Check sheet for the modelled part. Datum: model origin and axes. Units: mm. Face numbers are marked on the shaded views. A direction names the side the tool comes from. Coordinates: 2 decimals unless noted, no trailing zeros. Loops run counter-clockwise (first coordinate to the right, second up) from the corner with the lowest first, then second, coordinate; pieces in that order, holes last. Notation, with made-up numbers: (65, 29) - (121, 29) arc R29 ccw to (121, 56) - close; hole circle Ø9 at (75, 89). An arc over 180 degrees is marked (long way). Use a Markdown table: item, result. Add a question column.
1) Sectioned sample at C-C, the plane z = 11. Enter the section's corners in (x, y), then the cut area to 3 significant figures.
2) Tool access check on the marked faces 1, 2 and 3. Record the directions out of +Z, -Z, +X, -X, +Y, -Y that give a thin tool (end or side, any length) a straight path to the whole face; none if there is none.
3) Sectioned sample at A-A, the plane z = 0. Enter the section's corners in (x, y), then the cut area to 3 significant figures.
4) Sectioned sample at D-D, the plane z = -15. Enter the section's corners in (x, y).
5) Thickness scan on line 1 (X direction, y = 17, z = -5); line 2 (Z direction, x = 8.5, y = 17); line 3 (Y direction, x = 13.5, z = 1.5). Record the ranges inside material, lowest first.
6) Sectioned sample at B-B, the plane x = 13.5. Enter the section's corners in (y, z).
7) Go/stop test with flat-tipped pins: P1, Ø10, axis at x = 13, z = 8.5, coming from the +Y side; P2, Ø2, axis at x = 0, z = 10.5, coming from the -Y side; P3, Ø2, axis at x = 9.53, z = -5.5, coming from the -Y side. Record where each tip stops, or that it passes through.
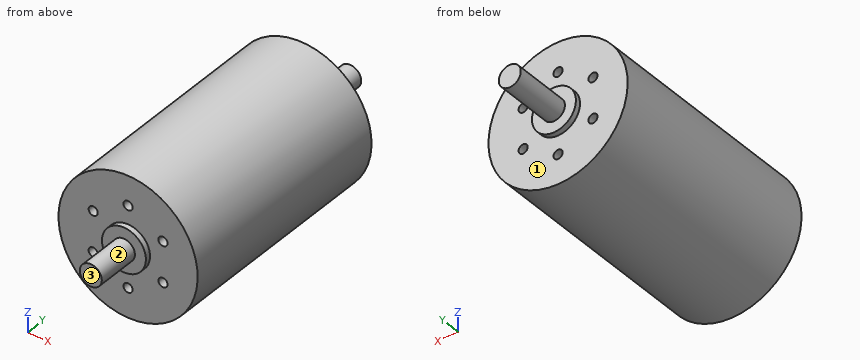
from build123d import *

# Parameters (mm, degrees)
ESQUISSE2_R             = 1.25
ENL_V_MAT_EXTRU_1_DEPTH = 5
ENL_V_START             = -58
ESQUISSE2_2_R           = 1.25
ENL_V_MAT_EXTRU_2_DEPTH = 5


with BuildPart() as part:
    # Esquisse1 → Révolution1 (revolve)
    with BuildSketch(Plane.XY, mode=Mode.PRIVATE) as r_volution1_sk:
        Polygon((0, 0), (0, 94), (3, 94), (3, 78), (6, 78), (6, 76.5), (19, 76.5), (19, 13.5), (6, 13.5), (6, 12), (3, 12), (3, 0), align=None)
    revolve(r_volution1_sk.sketch.rotate(Axis((0, 0, 0), (0, 1, 0)), 90), axis=Axis((0, 0, 0), (0, 1, 0)))

    # Esquisse2 → Enlèv. mat.-Extru.1 (cut)
    with BuildSketch(Plane(origin=(0, 76.5, 0), x_dir=(1, 0, 0), z_dir=(0, 1, 0))):
        with Locations(Location((0, 11, 0), (0, 0, 270))):
            Circle(ESQUISSE2_R)
        with Locations(Location((9.526279442, 5.5, 0), (0, 0, 270))):
            Circle(ESQUISSE2_R)
        with Locations(Location((9.526279442, -5.5, 0), (0, 0, 270))):
            Circle(ESQUISSE2_R)
        with Locations(Location((0, -11, 0), (0, 0, 270))):
            Circle(ESQUISSE2_R)
        with Locations(Location((-9.526279442, -5.5, 0), (0, 0, 270))):
            Circle(ESQUISSE2_R)
        with Locations(Location((-9.526279442, 5.5, 0), (0, 0, 270))):
            Circle(ESQUISSE2_R)
    extrude(amount=-ENL_V_MAT_EXTRU_1_DEPTH, mode=Mode.SUBTRACT)

    # Esquisse2<2> → Enlèv. mat.-Extru.2 (cut)
    with BuildSketch(Plane(origin=(0, 76.5, 0), x_dir=(1, 0, 0), z_dir=(0, 1, 0)).offset(ENL_V_START)):
        with Locations(Location((0, 11, 0), (0, 0, 270))):
            Circle(ESQUISSE2_2_R)
        with Locations(Location((9.526279442, 5.5, 0), (0, 0, 270))):
            Circle(ESQUISSE2_2_R)
        with Locations(Location((9.526279442, -5.5, 0), (0, 0, 270))):
            Circle(ESQUISSE2_2_R)
        with Locations(Location((0, -11, 0), (0, 0, 270))):
            Circle(ESQUISSE2_2_R)
        with Locations(Location((-9.526279442, -5.5, 0), (0, 0, 270))):
            Circle(ESQUISSE2_2_R)
        with Locations(Location((-9.526279442, 5.5, 0), (0, 0, 270))):
            Circle(ESQUISSE2_2_R)
    extrude(amount=-ENL_V_MAT_EXTRU_2_DEPTH, mode=Mode.SUBTRACT)


solid = part.part
Solved:
| question | item | result |
|---|---|---|
| 1 | outline | (-15.49, 13.5) - (-1.25, 13.5) - (-1.25, 18.5) - (1.25, 18.5) - (1.25, 13.5) - (15.49, 13.5) - (15.49, 76.5) - (1.25, 76.5) - (1.25, 71.5) - (-1.25, 71.5) - (-1.25, 76.5) - (-15.49, 76.5) - close |
| 1 | area | 1,930 mm2 |
| 2 | face 1 | +Y |
| 2 | face 2 | -Y |
| 2 | face 3 | +Z, -Z, +X, -X, -Y |
| 3 | outline | (-19, 13.5) - (-6, 13.5) - (-6, 12) - (-3, 12) - (-3, 0) - (3, 0) - (3, 12) - (6, 12) - (6, 13.5) - (19, 13.5) - (19, 76.5) - (6, 76.5) - (6, 78) - (3, 78) - (3, 94) - (-3, 94) - (-3, 78) - (-6, 78) - (-6, 76.5) - (-19, 76.5) - close |
| 3 | area | 2,600 mm2 |
| 4 | outline | (-11.66, 13.5) - (11.66, 13.5) - (11.66, 76.5) - (-11.66, 76.5) - close |
| 5 | line 1 | x = -18.33 to -10.67, -8.38 to 8.38, 10.67 to 18.33 |
| 5 | line 2 | z = -16.99 to -6.21, -4.79 to 4.79, 6.21 to 16.99 |
| 5 | line 3 | y = 13.5 to 76.5 |
| 6 | outline | (13.5, -13.37) - (76.5, -13.37) - (76.5, 13.37) - (13.5, 13.37) - close |
| 7 | P1 | stops at y = 76.5 |
| 7 | P2 | stops at y = 13.5 |
| 7 | P3 | stops at y = 18.5 |
